```python
from build123d import *

# Parameters (mm, degrees)
BOSS_EXTRUDE1_DEPTH       = 10
F_4_0MM_DOWEL_HOLE1_D     = 4
F_4_0MM_DOWEL_HOLE1_DEPTH = 10
F_4_0MM_DOWEL_HOLE1_TIP   = 1.201721238


with BuildPart() as part:
    # Sketch1 → Boss-Extrude1 (new body)
    with BuildSketch(Plane(origin=(0, 0, 0), x_dir=(0, 0, -1), z_dir=(1, 0, 0))):
        Polygon((-18.718400177, 4.62678414), (-8.598752597, 8), (-4.529205873, 8), (-4.529205873, 9.356515575), (42.401247403, 25), (42.401247403, 0), (-18.718400177, 0), align=None)
    extrude(amount=BOSS_EXTRUDE1_DEPTH)

    # Sketch9 → CSK for M4 Flat Head Machine Screw2 (revolve, cut)
    with BuildSketch(Plane(origin=(5, 8, 8.598752597), x_dir=(0, 0, 1), z_dir=(1, 0, 0))):
        Polygon((0, 0), (0, 11.351936393), (2.25, 10), (2.25, 2.45), (4.7, 0), align=None)
    revolve(axis=Axis((5, 14.35, 8.598752597), (0, -1, 0)), mode=Mode.SUBTRACT)

    # Ø4.0mm Dowel Hole1
    with Locations(Plane(origin=(5, 18, -42.401247403), x_dir=(0, -1, 0), z_dir=(0, 0, -1))):
        with Locations((0, 0), (11, 0)):
            Hole(F_4_0MM_DOWEL_HOLE1_D / 2, depth=F_4_0MM_DOWEL_HOLE1_DEPTH)
            with Locations((0, 0, -(F_4_0MM_DOWEL_HOLE1_DEPTH + F_4_0MM_DOWEL_HOLE1_TIP / 2))):  # 118° drill point
                Cone(0, F_4_0MM_DOWEL_HOLE1_D / 2, F_4_0MM_DOWEL_HOLE1_TIP, mode=Mode.SUBTRACT)


solid = part.part
```
Geometry check sheet. Reference: the model listing, model coordinates, mm. A direction names the side the tool comes from. Coordinates: 2 decimals unless noted, no trailing zeros. Loops run counter-clockwise (first coordinate to the right, second up) from the corner with the lowest first, then second, coordinate; pieces in that order, holes last.
Item 1: Go/stop test with flat-tipped pins: pin 1 Ø1.1 at (x, y) = (4.5, 9) entering from +Z; pin 2 Ø3 at (x, z) = (0.5, 6.5) entering from +Y; pin 3 Ø3 at (x, y) = (5, 7) entering from -Z. Record where each tip stops, or that it passes through.
Item 2: Release check for a two-part mould opening along X. For faces 1 (the face through (4.93, 17.07, -18.61)), 2 (the face through (0, 10, -19)), 3 (the face through (4.896, 6.669, -31.408)) record: released by +X, released by -X, zero draft, split by the parting line, or undercut.
Item 3: Sectioned sample at A-A, the plane z = -38. Record the boundary of the cut face in (x, y).
Item 4: Sectioned sample at B-B, the plane z = -16.5. Record the boundary of the cut face in (x, y), then the cut area to 3 significant figures.
Item 5: Thickness scan on line 1 (X direction, y = 7, z = -35.5); line 2 (Z direction, x = 5, y = 2.5); line 3 (X direction, y = 6.5, z = -38.5). Record the ranges inside material, lowest first.
Item 6: Sectioned sample at C-C, the plane z = 0. Record the boundary of the cut face in (x, y), then the cut area to 3 significant figures.
Item 7: Access from +Z, -Z, +X, -X, +Y, -Y to the whole of each face (thin tool, end or side, straight path). Record for faces 4 (the face through (6.2, 5.4, -37.3)), 5 (the face through (5, 13, -42.401)), 6 (the face through (0.7, 8, 5.7)).
Check result:
1. pin 1: stops at z = 4.53
1. pin 2: stops at y = 8
1. pin 3: stops at z = -32.1
2. face 1: zero draft
2. face 2: released by -X
2. face 3: undercut
3. outline: (0, 0) - (10, 0) - (10, 23.53) - (0, 23.53) - close; hole circle Ø4 at (5, 7); hole circle Ø4 at (5, 18)
4. outline: (0, 0) - (10, 0) - (10, 16.37) - (0, 16.37) - close
4. area: 164 mm2
5. line 1: x = 0 to 3, 7 to 10
5. line 2: z = -42.4 to 6.35, 10.85 to 18.72
5. line 3: x = 0 to 3.06, 6.94 to 10
6. outline: (0, 0) - (10, 0) - (10, 10.87) - (0, 10.87) - close
6. area: 109 mm2
7. face 4: -Z
7. face 5: -Z, +X, -X, +Y, -Y
7. face 6: +Z, +X, -X, +Y
